```python
from build123d import *

# Parameters (mm, degrees)
ESQUISSE1_R             = 1.5
ESQUISSE1_R_2           = 2
ESQUISSE1_R_3           = 4
BOSS_EXTRU_1_DEPTH      = 3
ESQUISSE4_R             = 2.563154281
ESQUISSE4_W             = 9.437600028
ESQUISSE4_H             = 17.69995175
BOSS_EXTRU_3_DEPTH      = 3
ESQUISSE5_R             = 1.5
ENL_V_MAT_EXTRU_1_DEPTH = 10
ESQUISSE6_R             = 1.5
BOSS_EXTRU_5_DEPTH      = 3
ESQUISSE7_R             = 1.5
ENL_V_MAT_EXTRU_2_DEPTH = 3
ESQUISSE8_R             = 1.5
ENL_V_MAT_EXTRU_3_DEPTH = 3
BOSS_EXTRU_7_DEPTH      = 3


with BuildPart() as part:
    # Esquisse1 → Boss.-Extru.1 (new body)
    with BuildSketch(Plane(origin=(0, 3, 0), x_dir=(1, 0, 0), z_dir=(0, 1, 0))):
        with BuildLine():
            Line((-24.441801488, 23.803313038), (-36.766762868, 4.367797016))
            ThreePointArc((-36.766762868, 4.367797016), (-36.940511073, 3.982727746), (-37, 3.564483978))
            Line((-37, 3.564483978), (-37, -3.639706512))
            ThreePointArc((-37, -3.639706512), (-36.958516169, -3.990035764), (-36.83635922, -4.320987683))
            Line((-36.83635922, -4.320987683), (-24.41738607, -28.681281171))
            ThreePointArc((-24.41738607, -28.681281171), (-23.864633333, -29.279046863), (-23.081026849, -29.5))
            Line((-23.081026849, -29.5), (-8.734084726, -29.5))
            ThreePointArc((-8.734084726, -29.5), (-8.074724869, -29.347310127), (-7.549601775, -28.920326105))
            Line((-7.549601775, -28.920326105), (7.477805006, -9.579673895))
            ThreePointArc((7.477805006, -9.579673895), (8.002928099, -9.152689873), (8.662287956, -9))
            Line((8.662287956, -9), (36.5, -9))
            ThreePointArc((36.5, -9), (37.560660172, -8.560660172), (38, -7.5))
            Line((38, -7.5), (38, 7.5))
            ThreePointArc((38, 7.5), (37.560660172, 8.560660172), (36.5, 9))
            Line((36.5, 9), (8.537585972, 9))
            ThreePointArc((8.537585972, 9), (7.973014245, 9.110302635), (7.491474184, 9.424988313))
            Line((7.491474184, 9.424988313), (-7.563270954, 24.075011687))
            ThreePointArc((-7.563270954, 24.075011687), (-8.044811015, 24.389697365), (-8.609382741, 24.5))
            Line((-8.609382741, 24.5), (-23.17503862, 24.5))
            ThreePointArc((-23.17503862, 24.5), (-23.897890764, 24.314338152), (-24.441801488, 23.803313038))
        make_face()
        with Locations(Location((33, -5, 0), (0, 0, 90))):
            Circle(ESQUISSE1_R, mode=Mode.SUBTRACT)
        with Locations(Location((-16, 12.5, 0), (0, 0, 90))):
            Circle(ESQUISSE1_R_2, mode=Mode.SUBTRACT)
        with Locations(Location((-21, -24.5, 0), (0, 0, 90))):
            Circle(ESQUISSE1_R, mode=Mode.SUBTRACT)
        with Locations(Location((-21, 19.5, 0), (0, 0, 90))):
            Circle(ESQUISSE1_R, mode=Mode.SUBTRACT)
        with Locations(Location((-16, -5, 0), (0, 0, 90))):
            Circle(ESQUISSE1_R, mode=Mode.SUBTRACT)
        with Locations(Location((-16, 5, 0), (0, 0, 90))):
            Circle(ESQUISSE1_R, mode=Mode.SUBTRACT)
        with Locations(Location((-11, 19.5, 0), (0, 0, 90))):
            Circle(ESQUISSE1_R, mode=Mode.SUBTRACT)
        with Locations(Location((-11, -24.5, 0), (0, 0, 90))):
            Circle(ESQUISSE1_R, mode=Mode.SUBTRACT)
        with Locations(Location((-32, 0, 0), (0, 0, 90))):
            Circle(ESQUISSE1_R, mode=Mode.SUBTRACT)
        with Locations(Location((-16, -13, 0), (0, 0, 90))):
            Circle(ESQUISSE1_R_3, mode=Mode.SUBTRACT)
        with Locations(Location((33, 5, 0), (0, 0, 90))):
            Circle(ESQUISSE1_R, mode=Mode.SUBTRACT)
        with BuildLine():
            Line((-26.75, -5), (-26.75, 5))
            ThreePointArc((-26.75, 5), (-26.017766953, 6.767766953), (-24.25, 7.5))
            Line((-24.25, 7.5), (-21.75, 7.5))
            ThreePointArc((-21.75, 7.5), (-19.982233047, 6.767766953), (-19.25, 5))
            Line((-19.25, 5), (-19.25, -5))
            ThreePointArc((-19.25, -5), (-19.982233047, -6.767766953), (-21.75, -7.5))
            Line((-21.75, -7.5), (-24.25, -7.5))
            ThreePointArc((-24.25, -7.5), (-26.017766953, -6.767766953), (-26.75, -5))
        make_face(mode=Mode.SUBTRACT)
        with BuildLine():
            Line((27.25, 2.5), (27.25, -2.5))
            ThreePointArc((27.25, -2.5), (26.810660172, -3.560660172), (25.75, -4))
            Line((25.75, -4), (7.745966692, -4))
            ThreePointArc((7.745966692, -4), (7.057719491, -4.167215025), (6.52291932, -4.631578947))
            ThreePointArc((6.52291932, -4.631578947), (-8, 0), (6.52291932, 4.631578947))
            ThreePointArc((6.52291932, 4.631578947), (7.057719491, 4.167215025), (7.745966692, 4))
            Line((7.745966692, 4), (25.75, 4))
            ThreePointArc((25.75, 4), (26.810660172, 3.560660172), (27.25, 2.5))
        make_face(mode=Mode.SUBTRACT)
    extrude(amount=-BOSS_EXTRU_1_DEPTH)

    # Esquisse4 → Boss.-Extru.3 (add)
    with BuildSketch(Plane(origin=(0, 3, 0), x_dir=(1, 0, 0), z_dir=(0, 1, 0))):
        with Locations((-32, 0)):
            Circle(ESQUISSE4_R)
        with BuildLine():
            Line((-8.428765835, 5.31043864), (-10.28347554, 5.31043864))
            Line((-10.28347554, 5.31043864), (-10.28347554, -6.18848711))
            Line((-10.28347554, -6.18848711), (-7.806886661, -6.18848711))
            ThreePointArc((-7.806886661, -6.18848711), (0, -9.96217105), (7.806886661, -6.18848711))
            Line((7.806886661, -6.18848711), (29.357557964, -6.18848711))
            Line((29.357557964, -6.18848711), (29.357557964, 5.31043864))
            Line((29.357557964, 5.31043864), (8.428765835, 5.31043864))
            ThreePointArc((8.428765835, 5.31043864), (0, 9.96217105), (-8.428765835, 5.31043864))
        make_face()
        with Locations((-22.804360287, -0.041920648)):
            Rectangle(ESQUISSE4_W, ESQUISSE4_H)
    extrude(amount=-BOSS_EXTRU_3_DEPTH)

    # Esquisse5 → Enlèv. mat.-Extru.1 (cut)
    with BuildSketch(Plane(origin=(0, 3, 0), x_dir=(1, 0, 0), z_dir=(0, 1, 0))):
        with Locations(Location((-30, 0, 0), (0, 0, 270))):
            Circle(ESQUISSE5_R)
        with BuildLine():
            Line((5.485812833, 4), (25.805812833, 4))
            Line((25.805812833, 4), (25.805812833, -4))
            Line((25.805812833, -4), (5.485812833, -4))
            ThreePointArc((5.485812833, -4), (4.797565631, -4.167215025), (4.26276546, -4.631578947))
            ThreePointArc((4.26276546, -4.631578947), (-10.26015386, 0), (4.26276546, 4.631578947))
            ThreePointArc((4.26276546, 4.631578947), (4.797565631, 4.167215025), (5.485812833, 4))
        make_face()
    extrude(amount=-ENL_V_MAT_EXTRU_1_DEPTH, mode=Mode.SUBTRACT)

    # Esquisse6 → Boss.-Extru.5 (add)
    with BuildSketch(Plane(origin=(0, 3, 0), x_dir=(1, 0, 0), z_dir=(0, 1, 0))):
        with Locations((33, 5)):
            Circle(ESQUISSE6_R)
        with Locations((33, -5)):
            Circle(ESQUISSE6_R)
    extrude(amount=-BOSS_EXTRU_5_DEPTH)

    # Esquisse7 → Enlèv. mat.-Extru.2 (cut)
    with BuildSketch(Plane(origin=(0, 3, 0), x_dir=(1, 0, 0), z_dir=(0, 1, 0))):
        with Locations(Location((31.975486082, 4.984695173, 0), (0, 0, 270))):
            Circle(ESQUISSE7_R)
        with Locations(Location((31.975486082, -5, 0), (0, 0, 270))):
            Circle(ESQUISSE7_R)
    extrude(amount=-ENL_V_MAT_EXTRU_2_DEPTH, mode=Mode.SUBTRACT)

    # Esquisse8 → Enlèv. mat.-Extru.3 (cut)
    with BuildSketch(Plane(origin=(0, 3, 0), x_dir=(1, 0, 0), z_dir=(0, 1, 0))):
        with Locations((-16.759449345, 5)):
            Circle(ESQUISSE8_R)
        with Locations((-16, 5)):
            Circle(ESQUISSE8_R)
        with Locations((-16.759449345, -5)):
            Circle(ESQUISSE8_R)
        with Locations((-16, -5)):
            Circle(ESQUISSE8_R)
    extrude(amount=-ENL_V_MAT_EXTRU_3_DEPTH, mode=Mode.SUBTRACT)

    # Esquisse10 → Boss.-Extru.7 (add)
    with BuildSketch(Plane(origin=(0, 3, 0), x_dir=(1, 0, 0), z_dir=(0, 1, 0))):
        with BuildLine():
            ThreePointArc((-16.379724673, 3.548859355), (-15.259449345, 5), (-16.379724673, 6.451140645))
            ThreePointArc((-16.379724673, 6.451140645), (-14.5, 5), (-16.379724673, 3.548859355))
        make_face()
        with BuildLine():
            ThreePointArc((-16.379724673, -6.451140645), (-15.259449345, -5), (-16.379724673, -3.548859355))
            ThreePointArc((-16.379724673, -3.548859355), (-14.5, -5), (-16.379724673, -6.451140645))
        make_face()
    extrude(amount=-BOSS_EXTRU_7_DEPTH)


solid = part.part
```
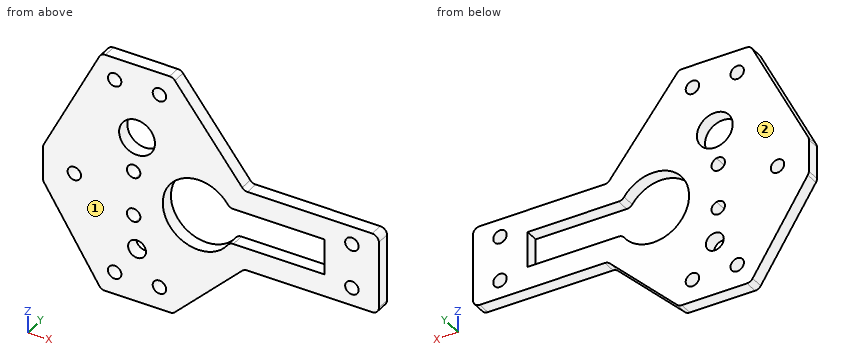
CAD build for the part. Positions are in the model's coordinates, mm. Face numbers are marked on the shaded views. Give positions to 0.01 mm unless a question says otherwise; leave off trailing zeros. Loops run counter-clockwise (first coordinate to the right, second up) from the corner with the lowest first, then second, coordinate; pieces in that order, holes last. Notation, with made-up numbers: M 52,87 L 83,87 A27 ccw 83,108 Z; hole C 88.5,59 d10. An arc over 180 degrees is marked long. Use one line per item in the form item = value.
Item 1: Slice it at B-B (z = 0). List the corners of the cut face in (x, y).
Determined:
outline = M -37,0 L -31.5,0 L -31.5,3 L -37,3 Z; M -28.5,0 L -10.26,0 L -10.26,3 L -28.5,3 Z; M 25.81,0 L 38,0 L 38,3 L 25.81,3 Z
Item 2: Slice it at C-C (z = -19.5). List the corners of the cut face in (x, y).
Determined:
outline = M -27.17,0 L -22.5,0 L -22.5,3 L -27.17,3 Z; M -19.5,0 L -12.5,0 L -12.5,3 L -19.5,3 Z; M -9.5,0 L -2.86,0 L -2.86,3 L -9.5,3 Z
Item 3: Flat gauge pins, fed straight in: pin 1 (1.8 mm diameter, centred on x = -16.76, z = 5, fed in from +Y); pin 2 (0.9 mm diameter, centred on x = 17.5, y = 1.5, fed in from +Z); pin 3 (1.5 mm diameter, centred on x = 23, y = 2, fed in from -Z). Where does each tip first touch, or does it go through?
Determined:
pin_1 = through
pin_2 = 9
pin_3 = -9
Item 4: Slice it at A-A (x = 20.5). List the corners of the cut face in (y, z).
Determined:
outline = M 0,-9 L 3,-9 L 3,-4 L 0,-4 Z; M 0,4 L 3,4 L 3,9 L 0,9 Z
Item 5: Two-plate mould, pull along Y, no slides. Class the marked faces 1 and 2: pulls with the +Y half, pulls with the -Y half, needs draft (parallel to the pull), parting line crosses it, or undercut.
Determined:
face_1 = pulls with the -Y half
face_2 = pulls with the +Y half
Item 6: Drill centre lines: probe 1 along Z at (x, y) = (-11, 1.1); probe 2 along Z at (x, y) = (15.5, 2.8); probe 3 along Z at (x, y) = (-22, 1.15). Where is each one in solid material? Low to high. Write a range as from..to.
Determined:
probe_1 = -24.5..-21, -18..23, 26..29.5
probe_2 = -9..-4, 4..9
probe_3 = -24.5..-20.62, -18.38..23.38, 25.62..29.5
Item 7: Slice it at D-D (y = 2.35). Count the separate pieces of the cut face and the enclosed holes in it, plus the area to 3 significant figures.
Determined:
separate_pieces = 1
enclosed_holes = 12
area = 1,890 mm2
